Geometry: final body of the model. Coordinates: model frame, mm. Face numbers are marked on the shaded views. A direction names the side the tool comes from. Coordinates: 2 decimals unless noted, no trailing zeros. Loops run counter-clockwise (first coordinate to the right, second up) from the corner with the lowest first, then second, coordinate; pieces in that order, holes last. Notation, with made-up numbers: (-31, -10.75) - (1, -10.75) arc R5 cw to (1, -4.75) - close; hole circle Ø3 at (-30.75, 60.5). An arc over 180 degrees is marked (long way). Answer in a Markdown table with one row per item.
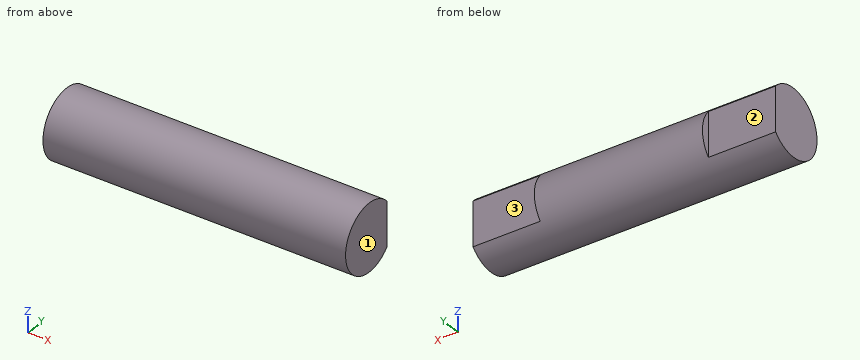
from build123d import *

# Parameters (mm, degrees)
SKETCH1_R           = 3.175
BOSS_EXTRUDE1_DEPTH = 28.575
SKETCH2_W           = 9.525
SKETCH2_H           = 1.5875
CUT_EXTRUDE1_DEPTH  = 6.35


with BuildPart() as part:
    # Sketch1 → Boss-Extrude1 (new body)
    with BuildSketch(Plane(origin=(0, 0, 0), x_dir=(0, 0, -1), z_dir=(1, 0, 0))):
        Circle(SKETCH1_R)
    extrude(amount=BOSS_EXTRUDE1_DEPTH)

    # Sketch2 → Cut-Extrude1 (cut)
    with BuildSketch(Plane(origin=(28.575, 0, 0), x_dir=(0, 0, -1), z_dir=(1, 0, 0))):
        with Locations((0, 3.175)):
            Rectangle(SKETCH2_W, SKETCH2_H)
    cut_extrude1 = extrude(amount=-CUT_EXTRUDE1_DEPTH, mode=Mode.SUBTRACT)

    # Mirror1: Cut-Extrude1 across plane
    add(cut_extrude1.mirror(Plane(origin=(14.2875, 0, 0), x_dir=(0, 0, 1), z_dir=(1, 0, 0))), mode=Mode.SUBTRACT)


solid = part.part
(1) Access query for the marked faces 1, 2 and 3. Directions: +Z, -Z, +X, -X, +Y, -Y. A direction counts if a zero-diameter tool reaches every point of the face in a straight line with its end or side. Return the directions, or none.
Verdict:
| item | result |
|---|---|
| face 1 | +Z, -Z, +X, +Y, -Y |
| face 2 | +Z, -Z, -X, +Y |
| face 3 | +Z, -Z, +X, +Y |
(2) First-contact query: pin 1 Ø0.6 at (y, z) = (3, -1) entering from -X; pin 2 Ø0.9 at (y, z) = (3, -0.5) entering from +X (3 decimals); pin 3 Ø2 at (x, z) = (26.5, 0.5) entering from +Y. Flat tips, straight axial feed; report the tip coordinate or a pass-through.
Verdict:
| item | result |
|---|---|
| pin 1 | stops at x = 6.35 |
| pin 2 | stops at x = 22.225 |
| pin 3 | stops at y = 2.38 |
(3) Cut plane D-D on x = 16. Output: boundary loops of the cut face in (y, z) (3 decimals), then the cut area to 3 significant figures.
Verdict:
| item | result |
|---|---|
| outline | circle Ø6.35 at (0, 0) |
| area | 31.7 mm² |
(4) Cut plane B-B on x = 27. Output: boundary loops of the cut face in (y, z) (3 decimals).
Verdict:
| item | result |
|---|---|
| outline | (2.381, -2.1) - (2.381, 2.1) arc R3.175 ccw (long way) to start |
(5) Cut plane C-C on y = 1.25. Output: boundary loops of the cut face in (x, z) (3 decimals), then the cut area to 3 significant figures.
Verdict:
| item | result |
|---|---|
| outline | (0, -2.919) - (28.575, -2.919) - (28.575, 2.919) - (0, 2.919) - close |
| area | 167 mm² |
(6) Cut plane A-A on z = 0. Output: boundary loops of the cut face in (x, y) (3 decimals).
Verdict:
| item | result |
|---|---|
| outline | (0, -3.175) - (28.575, -3.175) - (28.575, 2.381) - (22.225, 2.381) - (22.225, 3.175) - (6.35, 3.175) - (6.35, 2.381) - (0, 2.381) - close |
(7) Ray query, probe 1 along Z at (x, y) = (11.5, 2.25); probe 2 along Z at (x, y) = (7.5, -0.25); probe 3 along Y at (x, z) = (24, -0.5). Return the intervals inside material, ascending.
Verdict:
| item | result |
|---|---|
| probe 1 | z = -2.24 to 2.24 |
| probe 2 | z = -3.17 to 3.17 |
| probe 3 | y = -3.14 to 2.38 |
